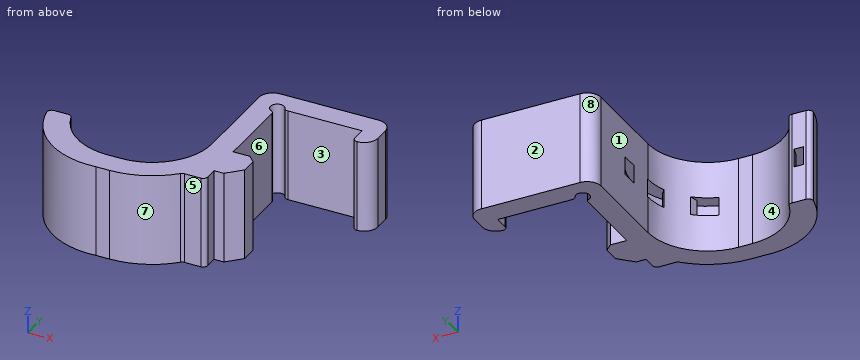
from build123d import *

# Parameters (mm, degrees)
BOSS_EXTRUDE1_DEPTH     = 20
FILLET1_R               = 3
CHAMFER1_SIZE           = 3
FILLET2_R               = 1
CUT_EXTRUDE1_DEPTH      = 2
CUT_EXTRUDE1_DEPTH_BACK = 2
CUT_EXTRUDE1_START      = -10
CHAMFER2_SIZE           = 1.5


with BuildPart() as part:
    # Sketch1 → Boss-Extrude1 (new body)
    with BuildSketch(Plane.XY):
        with BuildLine():
            Line((18, 45.5), (18, 41.407980081))
            Line((18, 41.407980081), (22, 41.407980081))
            Line((22, 41.407980081), (22, 50.5))
            Line((22, 50.5), (-5.5, 50.5))
            Line((-5.5, 50.5), (-5.5, 27.798635693))
            ThreePointArc((-5.5, 27.798635693), (-9.307611845, 18.606247538), (-18.5, 14.798635693))
            Line((-18.5, 14.798635693), (-21.5, 14.798635693))
            ThreePointArc((-21.5, 14.798635693), (-29.723519433, 17.585816031), (-34.557759664, 24.798635693))
            Line((-34.557759664, 24.798635693), (-39.557759664, 24.798635693))
            ThreePointArc((-39.557759664, 24.798635693), (-33.539294452, 13.674546113), (-21.5, 9.798635693))
            Line((-21.5, 9.798635693), (-18.5, 9.798635693))
            ThreePointArc((-18.5, 9.798635693), (-11.432404679, 11.244207392), (-5.5, 15.348736095))
            Line((-5.5, 15.348736095), (-0.5, 15.348736095))
            Line((-0.5, 15.348736095), (-0.5, 19))
            Line((-0.5, 19), (4.612884421, 19))
            Line((4.612884421, 19), (4.612884421, 27))
            Line((4.612884421, 27), (-0.5, 27))
            Line((-0.5, 27), (-0.5, 44))
            ThreePointArc((-0.5, 44), (-1.560660172, 46.560660172), (1, 45.5))
            Line((1, 45.5), (18, 45.5))
        make_face()
    extrude(amount=-BOSS_EXTRUDE1_DEPTH)

    # Fillet1
    fillet1_edges = [part.edges().sort_by_distance(p)[0] for p in [
        (-5.5, 50.5, -10),
        (22, 50.5, -10),
        (22, 41.407980081, -10),
    ]]
    fillet(fillet1_edges, radius=FILLET1_R)

    # Chamfer1
    chamfer1_edges = [part.edges().sort_by_distance(p)[0] for p in [
        (4.612884421, 19, -10),
    ]]
    chamfer(chamfer1_edges, length=CHAMFER1_SIZE)

    # Fillet2
    fillet2_edges = [part.edges().sort_by_distance(p)[0] for p in [
        (18, 41.407980081, -10),
        (-0.5, 15.348736095, -10),
        (-5.5, 15.348736095, -10),
        (-34.557759664, 24.798635693, -10),
        (-39.557759664, 24.798635693, -10),
        (-0.5, 44, -10),
        (1, 45.5, -10),
    ]]
    fillet(fillet2_edges, radius=FILLET2_R - 0.0001)  # a hair under: the kernel refuses the full size

    # Sketch3 → Cut-Extrude1 (cut, two sides: drawn at the far end of the back side and taken through both)
    with BuildSketch(Plane.XY.offset(CUT_EXTRUDE1_START - CUT_EXTRUDE1_DEPTH_BACK)):
        with BuildLine():
            Line((-18.5, 13.593483966), (-21.5, 13.593483966))
            ThreePointArc((-21.5, 13.593483966), (-30.584504262, 16.728345827), (-35.80235804, 24.798635693))
            Line((-35.80235804, 24.798635693), (-37.80235804, 24.798635693))
            ThreePointArc((-37.80235804, 24.798635693), (-31.973681851, 15.343278195), (-21.5, 11.644732532))
            Line((-21.5, 11.644732532), (-18.5, 11.644732532))
            ThreePointArc((-18.5, 11.644732532), (-4.080428513, 20.516840208), (-5.5, 37.387618296))
            Line((-5.5, 37.387618296), (-5.5, 33.524571041))
            ThreePointArc((-5.5, 33.524571041), (-4.487181784, 30.128284006), (-4.346617542, 26.586983672))
            ThreePointArc((-4.346617542, 26.586983672), (-4.771973785, 24.147932767), (-5.614362182, 21.819783493))
            ThreePointArc((-5.614362182, 21.819783493), (-7.568289903, 18.727580078), (-10.247050758, 16.236838064))
            ThreePointArc((-10.247050758, 16.236838064), (-12.457076385, 14.94292063), (-14.8635084, 14.066838125))
            ThreePointArc((-14.8635084, 14.066838125), (-16.666415033, 13.712319575), (-18.5, 13.593483966))
        make_face()
        with BuildLine():
            Line((-6.471563344, 22.867437906), (-5.614362182, 21.819783493))
            ThreePointArc((-5.614362182, 21.819783493), (-4.771973785, 24.147932767), (-4.346617542, 26.586983672))
            Line((-4.346617542, 26.586983672), (-5.5, 27.996625043))
            Line((-5.5, 27.996625043), (-5.5, 27.798635693))
            ThreePointArc((-5.5, 27.798635693), (-5.745203323, 25.285637139), (-6.471563344, 22.867437906))
        make_face()
        with BuildLine():
            Line((-14.54802471, 15.413891396), (-14.8635084, 14.066838125))
            ThreePointArc((-14.8635084, 14.066838125), (-12.457076385, 14.94292063), (-10.247050758, 16.236838064))
            Line((-10.247050758, 16.236838064), (-9.8019978, 18.137126612))
            ThreePointArc((-9.8019978, 18.137126612), (-12.030109342, 16.522975408), (-14.54802471, 15.413891396))
        make_face()
    extrude(amount=CUT_EXTRUDE1_DEPTH + CUT_EXTRUDE1_DEPTH_BACK, mode=Mode.SUBTRACT)

    # Chamfer2
    chamfer2_edges = [part.edges().sort_by_distance(p)[0] for p in [
        (4.612884421, 27, -10),
    ]]
    chamfer(chamfer2_edges, length=CHAMFER2_SIZE)


solid = part.part
Build history of the part. All positions in model axes, mm. Face numbers are marked on the shaded views. A direction names the side the tool comes from. Round coordinates to 2 decimals unless told otherwise and drop trailing zeros. Loops run counter-clockwise (first coordinate to the right, second up) from the corner with the lowest first, then second, coordinate; pieces in that order, holes last. Notation, with made-up numbers: (53.5, 67) -> (76.5, 67) arc R30 cw to (76.5, 102) -> close; hole circle Ø11 at (86.5, 23.25). An arc over 180 degrees is marked (long way). One line per item, written item: value. Start each with the question number.
Q1. Cut at A-A on y = 21. List the corners of the cut face in (x, z).
Q2. Cut at B-B on x = 4. List the corners of the cut face in (y, z), plus the area to 3 significant figures.
Q3. Two-plate mould, pull along Y, no slides. Class the marked faces 6, 7 and 8: released by +Y, released by -Y, zero draft, split by the parting line, or undercut.
Q4. Drop flat-ended pins along their axis: pin 1 Ø2.5 at (x, z) = (1, -7) entering from -Y; pin 2 Ø1 at (x, z) = (-30.5, -5) entering from -Y; pin 3 Ø3 at (y, z) = (18.5, -11.5) entering from +X; pin 4 Ø1.8 at (x, y) = (-0.5, 45.5) entering from -Z. Give the stop position or say it passes through.
Q5. Probe line 1 along Z through (x, y) = (-24, 13); line 2 along Y through (x, z) = (14, -10.75); line 3 along X through (y, z) = (22, -13.5). List the from-to ranges inside material, lowest first.
Q6. Cut at D-D on y = 31. List the corners of the cut face in (x, z), plus the area to 3 significant figures.
Q7. 3-axis set-ups, long thin cutter, end or side, ignore diameter. For the marked faces 1, 2, 3, 4 and 5: which of +Z, -Z, +X, -X, +Y, -Y reach the whole face in a straight line?
Computed:
1. outline: (-38.67, -20) -> (-32.87, -20) -> (-32.87, 0) -> (-38.67, 0) -> close; (-7.42, -20) -> (3.61, -20) -> (3.61, 0) -> (-7.42, 0) -> close; hole (-36.49, -12) -> (-34.28, -12) -> (-34.28, -8) -> (-36.49, -8) -> close; hole (-6.03, -12) -> (-3.85, -12) -> (-3.85, -8) -> (-6.03, -8) -> close
2. outline: (21.39, -20) -> (26.11, -20) -> (26.11, 0) -> (21.39, 0) -> close; (45.5, -20) -> (50.5, -20) -> (50.5, 0) -> (45.5, 0) -> close
2. area: 195 mm²
3. face 6: undercut
3. face 7: released by -Y
3. face 8: released by +Y
4. pin 1: y = 19
4. pin 2: y = 11.41
4. pin 3: x = 2.61
4. pin 4: through
5. line 1: -20 to -12, -8 to 0
5. line 2: 45.5 to 50.5
5. line 3: -39 to -33.46, -6.86 to 4.61
6. outline: (-5.5, -20) -> (-0.5, -20) -> (-0.5, 0) -> (-5.5, 0) -> close; hole (-4.66, -12) -> (-2.67, -12) -> (-2.67, -8) -> (-4.66, -8) -> close
6. area: 92.0 mm²
7. face 1: +Z, -Z, -X, +Y
7. face 2: +Z, -Z, +X, -X, +Y
7. face 3: +Z, -Z
7. face 4: +Z, -Z, +Y
7. face 5: +Z, -Z, +X, -Y
